Geometry: final body of the model. Coordinates: model frame, mm. Face numbers are marked on the shaded views. Give positions to 0.01 mm unless a question says otherwise; leave off trailing zeros. Write each loop counter-clockwise with the first axis right and the second up, starting at its lowest first coordinate (ties: lowest second). Pieces come first, ordered by that corner, then holes.
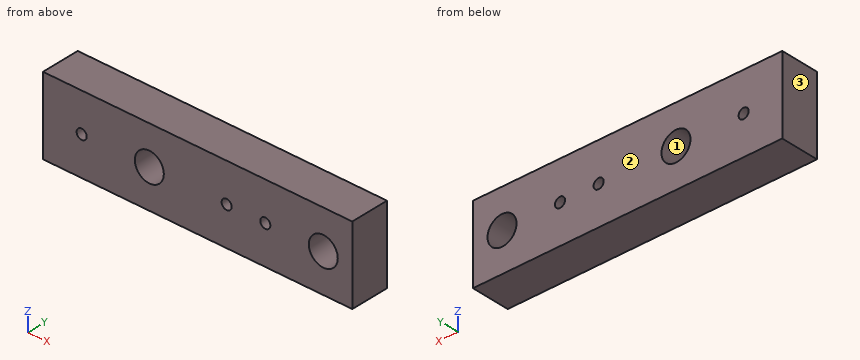
Autodesk Inventor part; units mm, degrees
ref_plane "YZ Plane" through (0, 0, 0) normal (1, 0, 0) x (0, 1, 0)
ref_plane "XZ Plane" through (0, 0, 0) normal (0, 1, 0) x (-1, 0, 0)
ref_plane "XY Plane" through (0, 0, 0) normal (0, 0, 1) x (1, 0, 0)
sketch "Sketch1" plane through (0, 0, 0) normal (1, 0, 0) x (0, 1, 0)
  line L0 (0, 0) -> (12.7, 0)
  line L1 (12.7, 0) -> (12.7, -25.4)
  line L2 (12.7, -25.4) -> (0, -25.4)
  line L3 (0, -25.4) -> (0, 0)
  dimension "d0" = 12.7
  dimension "d1" = 25.4
extrude "Extrusion1" add sketch "Sketch1" along normal blind 76.2
sketch "Sketch2" plane through (0, 12.7, 0) normal (0, 1, 0) x (1, 0, 0)
  circle A0 centre (9.525, 12.7) radius 4.7625
  line L0 (0, 0) -> (76.2, 0)
  line L1 (0, 25.4) -> (76.2, 25.4)
  line L2 (0, 0) -> (0, 25.4)
  circle A1 centre (66.675, 12.7) radius 4.7625
  line L3 (76.2, 25.4) -> (76.2, 0)
  dimension "d4" = 12.7
  dimension "d5" = 25.4
  dimension "d6" = 9.525
  dimension "d7" = 4.7625
  dimension "d8" = 9.525
  dimension "d9" = 12.7
  dimension "d10" = 4.7625
extrude "Extrusion2" cut sketch "Sketch2" against normal through all contours A0 | A1
sketch "Sketch5" plane through (0, 12.7, 0) normal (0, 1, 0) x (1, 0, 0)
  line L0 (0, 0) -> (76.2, 0)
  line L1 (0, 25.4) -> (76.2, 25.4)
  circle A0 centre (66.675, 12.7) radius 4.7625
  point P0 (47.625, 12.7)
  dimension "d26" = 12.7
  dimension "d27" = 25.4
  dimension "d28" = 19.05
hole "Hole2" at (47.625, 12.7, -12.7) direction (0, -1, 0) diameter 3.302 end through all
sketch "Sketch7" plane through (0, 0, 0) normal (-1, 0, 0) x (0, 0, 1)
  line L0 (-25.4, 12.7) -> (-25.4, 0)
  line L1 (0, 12.7) -> (-25.4, 12.7)
  line L2 (-25.4, 0) -> (0, 0)
  line L3 (0, 0) -> (0, 12.7)
  line L4 (0, 12.7) -> (-25.4, 12.7)
  line L5 (-25.4, 12.7) -> (-25.4, 0)
  point P0 (0, 0)
extrude "Extrusion4" add sketch "Sketch7" along normal blind 25.4
sketch "Sketch10" plane through (-25.4, 12.7, -25.4) normal (0, 1, 0) x (1, 0, 0)
  circle A0 centre (73.025, -12.7) radius 1.651
  circle A1 centre (34.925, -12.7) radius 4.7625
  circle A2 centre (92.075, -12.7) radius 4.7625
  line L0 (101.6, 0) -> (101.6, -25.4)
  line L1 (101.6, 0) -> (0, 0)
  line L2 (0, -25.4) -> (0, 0)
  line L3 (101.6, -25.4) -> (0, -25.4)
  point P0 (25.4, -25.4)
  point P1 (12.7, -12.7)
  point P2 (88.9, -38.1)
  dimension "d56" = 25.4
  dimension "d58" = 12.7
  dimension "d61" = 12.7
hole "Hole4" at (-12.7, 12.7, -12.7) at (63.5, 12.7, 12.7) direction (0, -1, 0) diameter 3.302 end through all
sketch "Sketch11" plane through (76.2, 12.7, 0) normal (0, 1, 0) x (1, 0, 0)
  circle A0 centre (-88.9, 12.7) radius 1.651
  circle A1 centre (-28.575, 12.7) radius 1.651
  circle A2 centre (-66.675, 12.7) radius 4.7625
  circle A3 centre (-9.525, 12.7) radius 4.7625
  line L0 (0, 0) -> (-101.6, 0)
  line L1 (0, 25.4) -> (0, 0)
  line L2 (0, 25.4) -> (-101.6, 25.4)
  line L3 (-101.6, 0) -> (-101.6, 25.4)
  point P0 (-76.2, 0)
  point P1 (-41.275, 12.7)
  dimension "d73" = 12.7
  dimension "d74" = 12.7
  dimension "d75" = 12.7
hole "Hole5" at (34.925, 12.7, -12.7) direction (0, -1, 0) diameter 3.302 end through all
equation "\"d4\" = 0.5 * d5"
equation "\"d8\" = d6"
equation "\"d9\" = d4"
equation "\"d10\" = d7"
properties part number "L17_TSI_004"
Q1. Section B-B on z = -12.7. Output: boundary loops of the cut face in (x, y).
Filled sheet:
outline: (-25.4, 0) - (-14.35, 0) - (-14.35, 12.7) - (-25.4, 12.7) - close; (-11.05, 0) - (4.76, 0) - (4.76, 12.7) - (-11.05, 12.7) - close; (14.29, 0) - (33.27, 0) - (33.27, 12.7) - (14.29, 12.7) - close; (36.58, 0) - (45.97, 0) - (45.97, 12.7) - (36.58, 12.7) - close; (49.28, 0) - (61.91, 0) - (61.91, 12.7) - (49.28, 12.7) - close; (71.44, 0) - (76.2, 0) - (76.2, 12.7) - (71.44, 12.7) - close
Q2. Section D-D on x = 9.5. Output: boundary loops of the cut face in (y, z).
Filled sheet:
outline: (0, -25.4) - (12.7, -25.4) - (12.7, -17.46) - (0, -17.46) - close; (0, -7.94) - (12.7, -7.94) - (12.7, 0) - (0, 0) - close
Q3. Pull-direction query (X, two-part tool) for the marked faces 1, 2 and 3; classes: released by +X, released by -X, zero draft, split by the parting line, or undercut.
Filled sheet:
face 1: undercut
face 2: zero draft
face 3: released by -X
Q4. Section C-C on y = 11.25. Output: boundary loops of the cut face in (x, z) (1 decimal), plus the area to 3 significant figures.
Filled sheet:
outline: (-25.4, -25.4) - (76.2, -25.4) - (76.2, 0) - (-25.4, 0) - close; hole circle Ø3.3 at (-12.7, -12.7); hole circle Ø9.5 at (9.5, -12.7); hole circle Ø3.3 at (34.9, -12.7); hole circle Ø3.3 at (47.6, -12.7); hole circle Ø9.5 at (66.7, -12.7)
area: 2,410 mm2
Q5. Ray query, line 1 along X through (y, z) = (9, -12.7); line 2 along X through (y, z) = (2, -10.25); line 3 along Z through (x, y) = (66, 7). Return the intervals inside material, ascending.
Filled sheet:
line 1: x = -25.4 to -14.35, -11.05 to 4.76, 14.29 to 33.27, 36.58 to 45.97, 49.28 to 61.91, 71.44 to 76.2
line 2: x = -25.4 to 5.44, 13.61 to 62.59, 70.76 to 76.2
line 3: z = -25.4 to -17.41, -7.99 to 0
Q6. Section A-A on x = -12.7. Output: boundary loops of the cut face in (y, z).
Filled sheet:
outline: (0, -25.4) - (12.7, -25.4) - (12.7, -14.35) - (0, -14.35) - close; (0, -11.05) - (12.7, -11.05) - (12.7, 0) - (0, 0) - close
Q7. Pin query (flat end, axial travel): P1, Ø3, axis at x = 47.625, z = -12.7, coming from the -Y side. Return the tip coordinate at first contact, or that it passes through.
Filled sheet:
P1: passes through
